Here's how the part is built. I have some questions about the finished solid (model axes, mm). Give positions to 0.01 mm unless a question says otherwise; leave off trailing zeros. Write each loop counter-clockwise with the first axis right and the second up, starting at its lowest first coordinate (ties: lowest second). Pieces come first, ordered by that corner, then holes. Notation, with made-up numbers: (3, 46.25) -> (38, 46.25) arc R28 ccw to (38, 64.25) -> close; hole circle Ø3 at (21, -14.5). An arc over 180 degrees is marked (long way). Return JSON: item names as keys, results as strings.
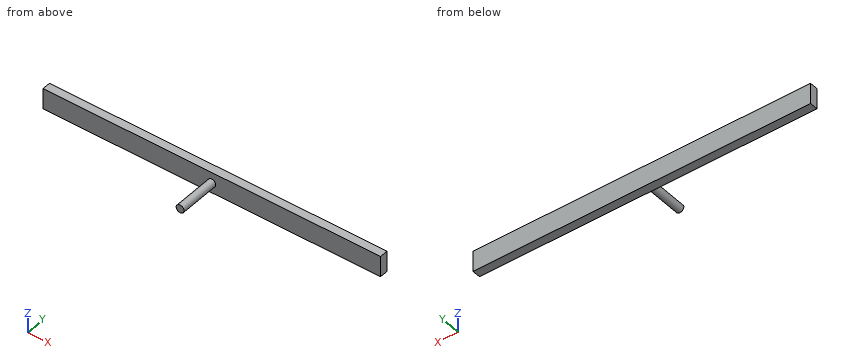
from build123d import *

# Parameters (mm, degrees)
SKETCH1_W           = 406.4
SKETCH1_H           = 10
BOSS_EXTRUDE1_DEPTH = 25
SKETCH2_R           = 4.75
BOSS_EXTRUDE2_DEPTH = 49


with BuildPart() as part:
    # Sketch1 → Boss-Extrude1 (new body)
    with BuildSketch(Plane.XY):
        with Locations((203.2, 5)):
            Rectangle(SKETCH1_W, SKETCH1_H)
    extrude(amount=BOSS_EXTRUDE1_DEPTH)

    # Sketch2 → Boss-Extrude2 (add)
    with BuildSketch(Plane.XZ):
        with Locations(Location((203.2, 12.25, 0), (0, 0, 90))):
            Circle(SKETCH2_R)
    extrude(amount=BOSS_EXTRUDE2_DEPTH)


solid = part.part
1. Suppose I cut it at A-A, the plane z = 12.25. List the corners of the cut face in (x, y) for me, and give its area (3 significant figures).
Taken from the geometry:
{"outline": "(0, 0) -> (198.45, 0) -> (198.45, -49) -> (207.95, -49) -> (207.95, 0) -> (406.4, 0) -> (406.4, 10) -> (0, 10) -> close", "area": "4,530 mm²"}
2. For pin 1 Ø4 at (x, z) = (352.5, 11.5) entering from -Y; pin 2 Ø1.5 at (y, z) = (-22, 16) entering from -X, each with a flat end and sliding along its axis, tell me the tip position at first contact or that it passes through.
Taken from the geometry:
{"pin 1": "stops at y = 0", "pin 2": "stops at x = 199.52"}
3. Suppose I cut it at C-C, the plane y = -38. List the corners of the cut face in (x, z) for me.
Taken from the geometry:
{"outline": "circle Ø9.5 at (203.2, 12.25)"}
4. Suppose I cut it at D-D, the plane x = 64. List the corners of the cut face in (y, z) for me.
Taken from the geometry:
{"outline": "(0, 0) -> (10, 0) -> (10, 25) -> (0, 25) -> close"}
5. Suppose I cut it at B-B, the plane x = 203.2. List the corners of the cut face in (y, z) for me, and give its area (4 significant figures).
Taken from the geometry:
{"outline": "(-49, 7.5) -> (0, 7.5) -> (0, 0) -> (10, 0) -> (10, 25) -> (0, 25) -> (0, 17) -> (-49, 17) -> close", "area": "715.5 mm²"}
6. If I drill on line 1 (Y direction, x = 185, z = 12.5); line 2 (X direction, y = -34, z = 11.5); line 3 (X direction, y = -23, z = 8.25), over which ranges is the centre line in solid material (lowest first)? Write a range as [from, to].
Taken from the geometry:
{"line 1": "y = [0, 10]", "line 2": "x = [198.51, 207.89]", "line 3": "x = [200.64, 205.76]"}
